```python
from build123d import *

# Parameters (mm, degrees)
ESTRUSIONE_ESTRUSIONE1_DEPTH = 3
SCHIZZO2_W                   = 20.66
SCHIZZO2_H                   = 13
ESTRUSIONE_ESTRUSIONE2_DEPTH = 14
TAGLIO_ESTRUSIONE1_DEPTH     = 25.91345219
SVUOTA1_T                    = -1
SCHIZZO4_R                   = 3.5
ESTRUSIONE_ESTRUSIONE3_DEPTH = 4
SCHIZZO5_R                   = 2.5
TAGLIO_ESTRUSIONE2_DEPTH     = 1
SCHIZZO6_R                   = 1.7
TAGLIO_ESTRUSIONE3_DEPTH     = 28.728326671
ESTRUSIONE_ESTRUSIONE4_DEPTH = 1.5
SCHIZZO8_R                   = 1.75
TAGLIO_ESTRUSIONE4_DEPTH     = 31.677517827
SCHIZZO9_R                   = 0.8
TAGLIO_ESTRUSIONE5_DEPTH     = 1.5
TAGLIO_ESTRUSIONE6_DEPTH     = 32.238759578
RACCORDO1_R                  = 1
SPECCHIA12_START             = 9
SPECCHIA12_DEPTH             = 1
RACCORDO2_R                  = 1
SPECCHIA15_START             = 9
SPECCHIA15_DEPTH             = 1
SCHIZZO12_R                  = 0.8
ESTRUSIONE_ESTRUSIONE5_DEPTH = 1.5
TAGLIO_ESTRUSIONE7_START     = -1
SCHIZZO13_R                  = 2.5
TAGLIO_ESTRUSIONE7_DEPTH     = 1


# Read off the part's stored shape, not the designer's step: Specchia12, Specchia15
with BuildPart() as part:
    # Schizzo1 → Estrusione-Estrusione1 (new body)
    with BuildSketch(Plane.XY):
        Polygon((-15.99, 4), (-10.33, 4), (-10.33, 10), (10.33, 10), (10.33, 4), (15.99, 4), (15.99, -3), (-15.99, -3), align=None)
    extrude(amount=ESTRUSIONE_ESTRUSIONE1_DEPTH)

    # Schizzo2 → Estrusione-Estrusione2 (add)
    with BuildSketch(Plane.XY):
        with Locations((0, 3.5)):
            Rectangle(SCHIZZO2_W, SCHIZZO2_H)
    extrude(amount=-ESTRUSIONE_ESTRUSIONE2_DEPTH)

    # Schizzo3 → Taglio-Estrusione1 (cut, through all)
    with BuildSketch(Plane(origin=(0, 10, 0), x_dir=(1, 0, 0), z_dir=(0, 1, 0))):
        Polygon((-10.33, 0), (-7.86142227, 14), (-10.33, 14), align=None)
    taglio_estrusione1 = extrude(amount=-TAGLIO_ESTRUSIONE1_DEPTH, mode=Mode.SUBTRACT)

    # Specchia1: Taglio-Estrusione1 across plane
    add(taglio_estrusione1.mirror(Plane(origin=(0, 0, 0), x_dir=(0, 0, 1), z_dir=(1, 0, 0))), mode=Mode.SUBTRACT)

    # Svuota1
    svuota1_openings = [part.faces().sort_by_distance(p)[0] for p in [
        (0, 2.81654304, 3),
    ]]
    offset(amount=SVUOTA1_T, openings=svuota1_openings, kind=Kind.INTERSECTION)

    # Schizzo4 → Estrusione-Estrusione3 (add)
    with BuildSketch(Plane.XY):
        with Locations(Location((-15.99, 0.5, 0), (0, 0, 270))):
            Circle(SCHIZZO4_R)
    estrusione_estrusione3 = extrude(amount=ESTRUSIONE_ESTRUSIONE3_DEPTH)

    # Schizzo5 → Taglio-Estrusione2 (cut)
    with BuildSketch(Plane.XY.offset(4)):
        with Locations((-15.99, 0.5)):
            Circle(SCHIZZO5_R)
    taglio_estrusione2 = extrude(amount=-TAGLIO_ESTRUSIONE2_DEPTH, mode=Mode.SUBTRACT)

    # Schizzo6 → Taglio-Estrusione3 (cut, through all)
    with BuildSketch(Plane.XY.offset(3)):
        with Locations((-15.99, 0.5)):
            Circle(SCHIZZO6_R)
    taglio_estrusione3 = extrude(amount=-TAGLIO_ESTRUSIONE3_DEPTH, mode=Mode.SUBTRACT)

    # Specchia2: Estrusione-Estrusione3, Taglio-Estrusione2, Taglio-Estrusione3 across plane
    add(estrusione_estrusione3.mirror(Plane(origin=(0, 0, 0), x_dir=(0, 0, 1), z_dir=(1, 0, 0))))
    add(taglio_estrusione2.mirror(Plane(origin=(0, 0, 0), x_dir=(0, 0, 1), z_dir=(1, 0, 0))), mode=Mode.SUBTRACT)
    add(taglio_estrusione3.mirror(Plane(origin=(0, 0, 0), x_dir=(0, 0, 1), z_dir=(1, 0, 0))), mode=Mode.SUBTRACT)

    # Schizzo7 → Estrusione-Estrusione4 (add)
    with BuildSketch(Plane(origin=(0, 0, -14), x_dir=(-1, 0, 0), z_dir=(0, 0, -1))):
        with BuildLine():
            Line((-7.86142227, 10), (-2.188751242, 16.051674439))
            ThreePointArc((-2.188751242, 16.051674439), (0, 17), (2.188751242, 16.051674439))
            Line((2.188751242, 16.051674439), (7.86142227, 10))
            Line((7.86142227, 10), (-7.86142227, 10))
        make_face()
    extrude(amount=-ESTRUSIONE_ESTRUSIONE4_DEPTH)

    # Schizzo8 → Taglio-Estrusione4 (cut, through all)
    with BuildSketch(Plane.XY.offset(-12.5)):
        with Locations((0, 14)):
            Circle(SCHIZZO8_R)
    extrude(amount=-TAGLIO_ESTRUSIONE4_DEPTH, mode=Mode.SUBTRACT)

    # Schizzo9 → Taglio-Estrusione5 (cut)
    with BuildSketch(Plane(origin=(0, 0, -14), x_dir=(-1, 0, 0), z_dir=(0, 0, -1))):
        with Locations((-5.36142227, 7.5)):
            Circle(SCHIZZO9_R)
    taglio_estrusione5 = extrude(amount=-TAGLIO_ESTRUSIONE5_DEPTH, mode=Mode.SUBTRACT)

    # Specchia5: Taglio-Estrusione5 across plane
    add(taglio_estrusione5.mirror(Plane(origin=(0, 0, 0), x_dir=(0, 0, 1), z_dir=(1, 0, 0))), mode=Mode.SUBTRACT)

    # Schizzo10 → Taglio-Estrusione6 (cut, through all)
    with BuildSketch(Plane.XZ.offset(3)):
        Polygon((-6.289561189, 3), (-4.17363742, -9), (4.17363742, -9), (6.289561189, 3), align=None)
    extrude(amount=-TAGLIO_ESTRUSIONE6_DEPTH, mode=Mode.SUBTRACT)

    # Raccordo1
    raccordo1_edges = [part.edges().sort_by_distance(p)[0] for p in [
        (-4.17363742, -2.5, -9),
    ]]
    fillet(raccordo1_edges, radius=RACCORDO1_R)

    # Specchia12 outline → Specchia12 (add)
    with BuildSketch(Plane(origin=(0, 0, 0), x_dir=(1, 0, 0), z_dir=(0, 1, 0)).offset(SPECCHIA12_START)):
        with BuildLine():
            ThreePointArc((-4.319345542, 8.173648178), (-3.977325399, 8.766044443), (-3.334537789, 9))
            Line((-3.334537789, 9), (-4.17363742, 9))
            Line((-4.17363742, 9), (-4.319345542, 8.173648178))
        make_face()
    extrude(amount=SPECCHIA12_DEPTH)

    # Raccordo2
    raccordo2_edges = [part.edges().sort_by_distance(p)[0] for p in [
        (4.17363742, -2.5, -9),
    ]]
    fillet(raccordo2_edges, radius=RACCORDO2_R)

    # Specchia15 outline → Specchia15 (add)
    with BuildSketch(Plane(origin=(0, 0, 0), x_dir=(1, 0, 0), z_dir=(0, 1, 0)).offset(SPECCHIA15_START)):
        with BuildLine():
            ThreePointArc((3.334537789, 9), (3.977325399, 8.766044443), (4.319345542, 8.173648178))
            Line((4.319345542, 8.173648178), (4.17363742, 9))
            Line((4.17363742, 9), (3.334537789, 9))
        make_face()
    extrude(amount=SPECCHIA15_DEPTH)

    # Schizzo12 → Estrusione-Estrusione5 (add)
    with BuildSketch(Plane(origin=(0, 0, -14), x_dir=(-1, 0, 0), z_dir=(0, 0, -1))):
        with BuildLine():
            Line((-7.86142227, -3), (-2.188751242, -9.051674439))
            ThreePointArc((-2.188751242, -9.051674439), (0, -10), (2.188751242, -9.051674439))
            Line((2.188751242, -9.051674439), (7.86142227, -3))
            Line((7.86142227, -3), (-7.86142227, -3))
        make_face()
        with Locations((0, -4.5)):
            Circle(SCHIZZO12_R, mode=Mode.SUBTRACT)
    extrude(amount=-ESTRUSIONE_ESTRUSIONE5_DEPTH)

    # Schizzo13 → Taglio-Estrusione7 (cut)
    with BuildSketch(Plane(origin=(0, 0, 0), x_dir=(-1, 0, 0), z_dir=(0, 0, -1)).offset(TAGLIO_ESTRUSIONE7_START)):
        with Locations((-15.99, 0.5)):
            Circle(SCHIZZO13_R)
    taglio_estrusione7 = extrude(amount=TAGLIO_ESTRUSIONE7_DEPTH, mode=Mode.SUBTRACT)

    # Specchia16: Taglio-Estrusione7 across plane
    add(taglio_estrusione7.mirror(Plane(origin=(0, 0, 0), x_dir=(0, 0, 1), z_dir=(1, 0, 0))), mode=Mode.SUBTRACT)


solid = part.part
```
Verification items for the finished model (mm, model axes). A direction names the side the tool comes from. Round coordinates to 2 decimals unless told otherwise and drop trailing zeros. Order: outer loops, then holes, each group sorted by start corner. A loop starts at its lowest first (then second) coordinate and runs counter-clockwise, first axis right, second up. Notation, with made-up numbers: (25, -6) -> (29, -6) arc R23 cw to (29, 30) -> close; hole circle Ø5 at (35.5, -22.75). An arc over 180 degrees is marked (long way). Put each result on its own line as item: value. Start each with the question number.
(1) Section check A-A (x = 0). Enter the section's corners in (y, z), then the cut area to 4 significant figures.
(2) Section check C-C (z = -3). Enter the section's corners in (x, y), then the cut area to 3 significant figures.
(3) Material ranges on line 1 along Y through (x, z) = (0, -13.6); line 2 along X through (y, z) = (5.5, 1.5); line 3 along Y through (x, z) = (9, 0.5), recorded low to high.
(4) Section check B-B (y = 7.5). Enter the section's corners in (x, z).
(5) Draft check along Y on faces 1 (the face through (-19.095, -1.115, 2.416)), 2 (the face through (-0.1, 10, -9.4)), 3 (the face through (15, 3, 4)). Enter one of: +Y half, -Y half, draft (parallel to the pull), parting line (faces both ways), or undercut.
(6) Tool access check on faces 4 (the face through (13, 1, 0)), 5 (the face through (0, 12, -12.5)), 6 (the face through (3.97, -2.49, -8.77)), 7 (the face through (0, -6, -12.5)), 8 (the face through (18.488, 0.61, 3.507)). Record the directions out of +Z, -Z, +X, -X, +Y, -Y that give a thin tool (end or side, any length) a straight path to the whole face; none if there is none.
(7) Depth check by flat-ended pin: pin 1 Ø1.8 at (x, y) = (0, -4.5) entering from +Z; pin 2 Ø1.5 at (x, y) = (-15, 0) entering from -Z; pin 3 Ø10 at (y, z) = (-6.5, -5) entering from +X. Enter the tip coordinate at first touch or a pass-through.
(8) Section check D-D (y = -4.5). Enter the section's corners in (x, z), then the cut area to 3 significant figures.
Completed:
1. outline: (-10, -14) -> (-5.3, -14) -> (-5.3, -12.5) -> (-10, -12.5) -> close; (-3.7, -14) -> (12.25, -14) -> (12.25, -12.5) -> (10, -12.5) -> (10, -9) -> (9, -9) -> (9, -13) -> (-2, -13) -> (-2, -9) -> (-3, -9) -> (-3, -12.5) -> (-3.7, -12.5) -> close; (15.75, -14) -> (17, -14) -> (17, -12.5) -> (15.75, -12.5) -> close
1. area: 34.35 mm2
2. outline: (-9.8, -3) -> (-5.23, -3) -> (-5.23, -2) -> (-8.79, -2) -> (-8.79, 9) -> (-5.23, 9) -> (-5.23, 10) -> (-9.8, 10) -> close; (5.23, -3) -> (9.8, -3) -> (9.8, 10) -> (5.23, 10) -> (5.23, 9) -> (8.79, 9) -> (8.79, -2) -> (5.23, -2) -> close
2. area: 40.6 mm2
3. line 1: y = -10 to -5.3, -3.7 to 12.25, 15.75 to 17
3. line 2: x = -10.33 to -9.33, 9.33 to 10.33
3. line 3: y = -3 to -2, 9 to 10
4. outline: (-10.33, 0) -> (-7.86, -14) -> (-6.16, -14) -> (-6.16, -13) -> (-7.02, -13) -> (-9.33, 0.09) -> (-9.33, 3) -> (-10.33, 3) -> close; (-4.56, -14) -> (4.56, -14) -> (4.56, -13) -> (-4.56, -13) -> close; (6.16, -14) -> (7.86, -14) -> (10.33, 0) -> (10.33, 3) -> (9.33, 3) -> (9.33, 0.09) -> (7.02, -13) -> (6.16, -13) -> close
5. face 1: undercut
5. face 2: +Y half
5. face 3: draft
6. face 4: -Z, +X, +Y, -Y
6. face 5: +Z, +X, -X, +Y
6. face 6: +Z, +Y, -Y
6. face 7: +Z, +X, -X, -Y
6. face 8: +Z
7. pin 1: stops at z = -12.5
7. pin 2: stops at z = 1
7. pin 3: stops at x = 10.08
8. outline: (-6.46, -14) -> (-0.8, -14) -> (-0.8, -12.5) -> (-6.46, -12.5) -> close; (0.8, -14) -> (6.46, -14) -> (6.46, -12.5) -> (0.8, -12.5) -> close
8. area: 17.0 mm2
